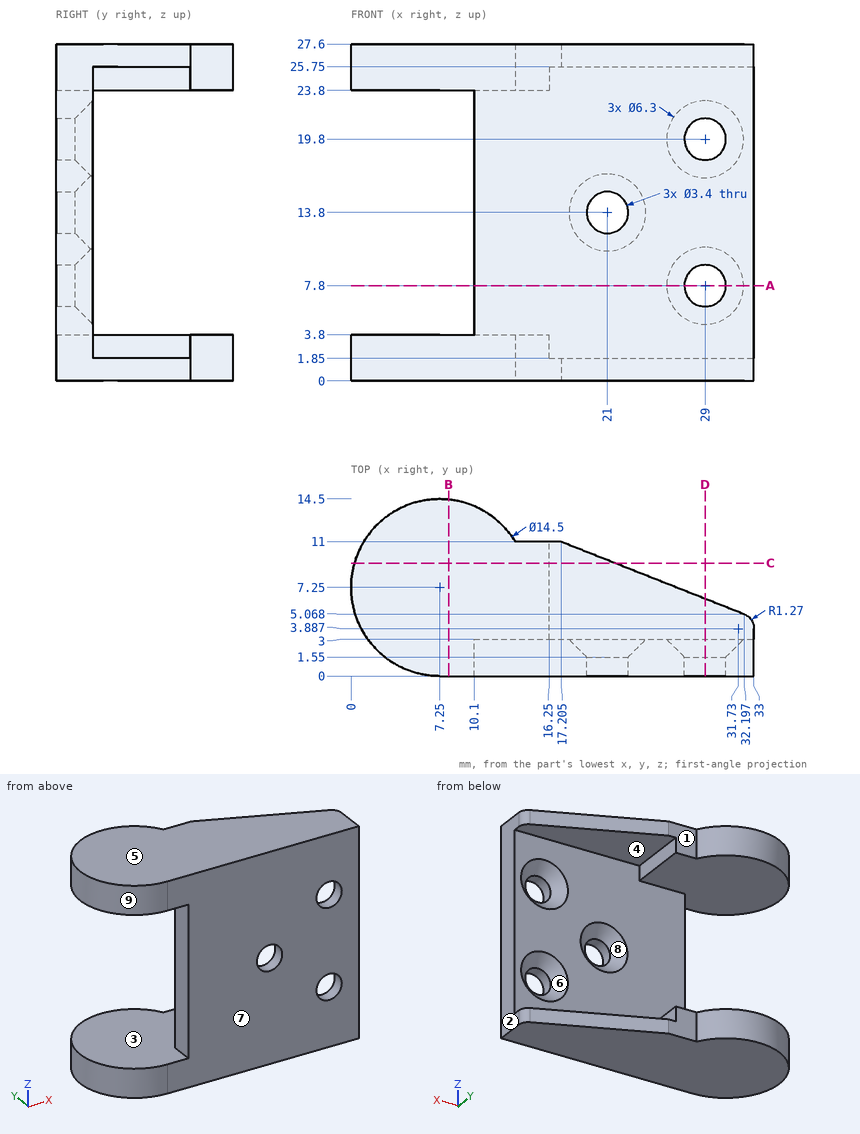
Check sheet for the drawn part. Datum: minimum x, y, z corner. Units: mm. A direction names the side the tool comes from. Round coordinates to 2 decimals unless told otherwise and drop trailing zeros. Loops run counter-clockwise (first coordinate to the right, second up) from the corner with the lowest first, then second, coordinate; pieces in that order, holes last. Notation, with made-up numbers: M 83.5,53.25 L 120.5,53.25 A25 cw 120.5,69.25 Z; hole C -29,-2.5 d2. An arc over 180 degrees is marked long. One line per question, with ' | ' between items. Start each with the question number.
Item 1: Section check A-A (z = 7.8). Record the boundary of the cut face in (x, y).
Item 2: Scan lines: probe 1 along Z at (x, y) = (29, 0.85); probe 2 along X at (y, z) = (1.15, 13.8); probe 3 along X at (y, z) = (0.8, 7.8). Record each from-to range of solid material in increasing order.
Item 3: Release check for a two-part mould opening along X. For the marked faces 6, 7, 8 and 9 record: released by +X, released by -X, zero draft, split by the parting line, or undercut.
Item 4: Section check B-B (x = 8). Record the boundary of the cut face in (y, z).
Item 5: Set-up check for the marked faces 1, 2, 3, 4 and 5: record each of +Z, -Z, +X, -X, +Y, -Y from which the full face is reachable in a straight line by a thin tool's end or side.
Item 6: Gauge pin test, flat ends, axial feed: pin 1 Ø1.6 at (y, z) = (5, 3) entering from +X; pin 2 Ø2 at (y, z) = (12.5, 22.5) entering from -X; pin 3 Ø0.9 at (y, z) = (1, 16) entering from -X; pin 4 Ø1.9 at (x, z) = (15.5, 3) entering from +Y. Record the tip position at first contact, or that the pin passes through.
Item 7: Section check C-C (y = 9.25). Record the boundary of the cut face in (x, z), and give its area (3 significant figures).
Item 8: Section check D-D (x = 29). Record the boundary of the cut face in (y, z).
Worked out:
1) outline: M 10.1,0 L 27.3,0 L 27.3,1.55 L 25.85,3 L 10.1,3 Z; M 30.7,0 L 33,0 L 33,3 L 32.15,3 L 30.7,1.55 Z
2) probe 1: 0 to 6.1, 9.5 to 18.1, 21.5 to 27.6 | probe 2: 10.1 to 19.3, 22.7 to 33 | probe 3: 10.1 to 27.3, 30.7 to 33
3) face 6: undercut | face 7: zero draft | face 8: undercut | face 9: split by the parting line
4) outline: M 0,0 L 14.46,0 L 14.46,3.8 L 0,3.8 Z; M 0,23.8 L 14.46,23.8 L 14.46,27.6 L 0,27.6 Z
5) face 1: +Z, -Z, +X, +Y | face 2: +Z, -Z, +X, +Y, -Y | face 3: -X, +Y | face 4: +X, +Y | face 5: +Z, +X, -X, +Y, -Y
6) pin 1: x = 16.25 | pin 2: through | pin 3: x = 10.1 | pin 4: y = 11
7) outline: M 0.28,0 L 21.63,0 L 21.63,1.85 L 16.25,1.85 L 16.25,3.8 L 0.28,3.8 Z; M 0.28,23.8 L 16.25,23.8 L 16.25,25.75 L 21.63,25.75 L 21.63,27.6 L 0.28,27.6 Z | area: 141 mm^2
8) outline: M 0,0 L 6.33,0 L 6.33,1.85 L 3,1.85 L 3,4.65 L 1.55,6.1 L 0,6.1 Z; M 0,9.5 L 1.55,9.5 L 3,10.95 L 3,16.65 L 1.55,18.1 L 0,18.1 Z; M 0,21.5 L 1.55,21.5 L 3,22.95 L 3,25.75 L 6.33,25.75 L 6.33,27.6 L 0,27.6 Z
